The listing builds one solid part. Answer for the finished solid, in the listing's coordinates (mm). Face numbers are marked on the shaded views. A direction names the side the tool comes from. Give positions to 0.01 mm unless a question says otherwise; leave off trailing zeros. Order: outer loops, then holes, each group sorted by start corner. A loop starts at its lowest first (then second) coordinate and runs counter-clockwise, first axis right, second up. Notation, with made-up numbers: (31, 28) - (57, 28) arc R7 cw to (57, 37) - close; hole circle Ø10 at (2.5, 68.5). An arc over 180 degrees is marked (long way). Answer in a Markdown table with one row per item.
from build123d import *

# Parameters (mm, degrees)
BOSS_EXTRUDE1_DEPTH = 7.1374
SKETCH2_W           = 4.5
SKETCH2_H           = 4.5
BOSS_EXTRUDE2_DEPTH = 3


with BuildPart() as part:
    # Sketch1 → Boss-Extrude1 (new body)
    with BuildSketch(Plane.XY):
        with BuildLine():
            Line((0, 0), (0, -12.7))
            Line((0, -12.7), (9.23036, -12.7))
            Line((9.23036, -12.7), (9.23036, 0))
            ThreePointArc((9.23036, 0), (7.937079259, 3.18640613), (4.788897173, 4.570136108))
            Line((4.788897173, 4.570136108), (4.441462827, 4.570136108))
            ThreePointArc((4.441462827, 4.570136108), (1.293280741, 3.18640613), (0, 0))
        make_face()
    extrude(amount=BOSS_EXTRUDE1_DEPTH)

    # Sketch2 → Boss-Extrude2 (add)
    with BuildSketch(Plane.XZ.offset(12.7)):
        with Locations((4.61518, 3.5687)):
            Rectangle(SKETCH2_W, SKETCH2_H)
    extrude(amount=BOSS_EXTRUDE2_DEPTH)


solid = part.part
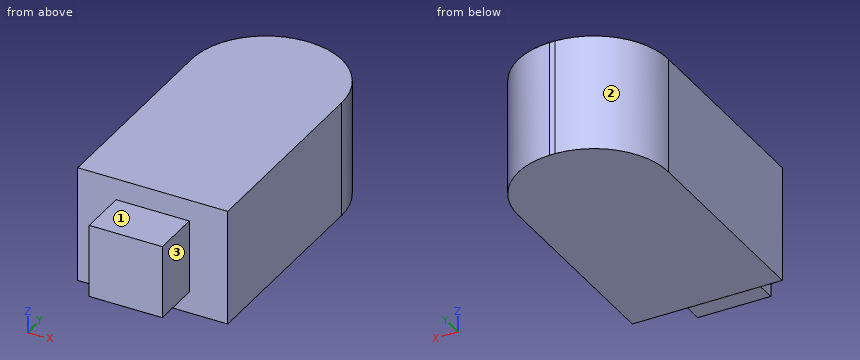
Item 1: Find section D-D on z = 6.5. Write down the section's boundary in (x, y).
Answer block:
| item | result |
|---|---|
| outline | (0, -12.7) - (9.23, -12.7) - (9.23, 0) arc R4.57 ccw to (4.79, 4.57) - (4.44, 4.57) arc R4.57 ccw to (0, 0) - close |
Item 2: Consider line 1 (X direction, y = -12.75, z = 1.75); line 2 (Y direction, x = 3.5, z = 1.25); line 3 (X direction, y = 3.25, z = 2.5). Determine where each line is inside the solid, lowest interval first.
Answer block:
| item | result |
|---|---|
| line 1 | 2.37 to 6.87 |
| line 2 | -12.7 to 4.44 |
| line 3 | 1.36 to 7.87 |
Item 3: Find section A-A on z = 2.5. Write down the section's boundary in (x, y), then the cut area to 3 significant figures.
Answer block:
| item | result |
|---|---|
| outline | (0, -12.7) - (2.37, -12.7) - (2.37, -15.7) - (6.87, -15.7) - (6.87, -12.7) - (9.23, -12.7) - (9.23, 0) arc R4.57 ccw to (4.79, 4.57) - (4.44, 4.57) arc R4.57 ccw to (0, 0) - close |
| area | 164 mm² |
Item 4: Each of these flat-tipped pins is pushed along its axis until it touches: P1, Ø1.5, axis at x = 5.5, y = -13.5, coming from the -Z side; P2, Ø2.5, axis at y = -14, z = 2.5, coming from the +X side; P3, Ø1.5, axis at x = 4.5, y = -13.5, coming from the +Z side. Where does it stop, or does it pass through?
Answer block:
| item | result |
|---|---|
| P1 | z = 1.32 |
| P2 | x = 6.87 |
| P3 | z = 5.82 |
Item 5: Which of the six approach directions +Z, -Z, +X, -X, +Y, -Y give full straight-line access (tool end or side, diameter ignored) to the marked faces 1, 2 and 3?
Answer block:
| item | result |
|---|---|
| face 1 | +Z, +X, -X, -Y |
| face 2 | +Z, -Z, -X, +Y |
| face 3 | +Z, -Z, +X, -Y |
Item 6: Find section C-C on y = -13.5. Write down the section's boundary in (x, z).
Answer block:
| item | result |
|---|---|
| outline | (2.37, 1.32) - (6.87, 1.32) - (6.87, 5.82) - (2.37, 5.82) - close |
Item 7: Find section B-B on x = 3.75. Write down the section's boundary in (y, z), then the cut area to 3 significant figures.
Answer block:
| item | result |
|---|---|
| outline | (-15.7, 1.32) - (-12.7, 1.32) - (-12.7, 0) - (4.5, 0) - (4.5, 7.14) - (-12.7, 7.14) - (-12.7, 5.82) - (-15.7, 5.82) - close |
| area | 136 mm² |
